The model under review builds one solid part; all positions refer to its coordinate system, in mm. Give positions to 0.01 mm unless a question says otherwise; leave off trailing zeros. Write each question's results on one line, items separated by ' | '. Start each with the question number.
Q1. Insertion check: pin 1 Ø1.3 at (x, z) = (3.5, -2.5) entering from +Y; pin 2 Ø6 at (x, z) = (7.5, 4.5) entering from -Y; pin 3 Ø1 at (x, z) = (-18, -8.5) entering from -Y. Each pin has a flat end and moves straight along its axis. Give the tip position at first contact, or say it passes through.
Q2. Wall thickness on L1, parallel to Y at x = -15.5, z = 5.5; L2, parallel to Y at x = -8, z = -5.75: over which ranges is each line inside the solid? List them lowest first. Write a range as [from, to].
Q3. Mouldability with a two-part tool opening along Z and no side actions: class faces 1 (the face through (16.507, 0.507, 8.229)), 2 (the face through (-15, 8, -4)), 3 (the face through (0, 4, 9.5)) as released by +Z, released by -Z, zero draft, split by the parting line, or undercut.
from build123d import *

# Parameters (mm, degrees)
SKETCH_1_W             = 37.6
SKETCH_1_H             = 19
EXTRUDE_1_DEPTH        = 8.1
SKETCH_3_R             = 0.75
CUT_EXTRUDE_1_DEPTH    = 0.1
PATTERN_LINEAR_1_COUNT = 3
PATTERN_LINEAR_1_PITCH = 12.7
CUT_EXTRUDE_4_DEPTH    = 28.929375217
CUT_EXTRUDE_5_DEPTH    = 40.618430055
EXTRUDE_3_DEPTH        = 2.5
EXTRUDE_3_DEPTH_BACK   = 1
SKETCH_7_R             = 0.25


with BuildPart() as part:
    # Эскиз1 → Бобышка-Вытянуть1 (new body)
    with BuildSketch(Plane(origin=(0, 0, 0), x_dir=(1, 0, 0), z_dir=(0, 1, 0))):
        Rectangle(SKETCH_1_W, SKETCH_1_H)
    extrude(amount=EXTRUDE_1_DEPTH)

    # Эскиз3 → Вырез-Вытянуть1 (cut)
    with BuildSketch(Plane(origin=(0, 8.1, 0), x_dir=(1, 0, 0), z_dir=(0, 1, 0))):
        with Locations(Location((-8.304984536, -7.1, 0), (0, 0, 270))):
            Circle(SKETCH_3_R)
        with BuildLine():
            Line((-16.613732692, -0.2), (-15.694010352, -0.2))
            Line((-15.694010352, -0.2), (-15.219253427, -0.887312434))
            Line((-15.219253427, -0.887312434), (-16.426812093, -7.1))
            Line((-16.426812093, -7.1), (-16.741799663, -7.1))
            ThreePointArc((-16.741799663, -7.1), (-17.513421017, -6.736082138), (-17.723428784, -5.909200972))
            Line((-17.723428784, -5.909200972), (-16.613732692, -0.2))
        make_face()
        Polygon((-15.447560185, -0.028936325), (-14.606711256, 0.75), (-10.084601751, 0.75), (-9.951753914, 0.611535824), (-9.389365278, 0.025371374), (-10.434703803, -0.75), (-14.949489793, -0.75), align=None)
        Polygon((-13.658315987, 5.6), (-13.366761329, 7.1), (-8.873187907, 7.1), (-9.164742565, 5.6), align=None)
        Polygon((-16.126812093, -7.1), (-15.835257435, -5.6), (-11.341684013, -5.6), (-11.633238671, -7.1), align=None)
        with BuildLine():
            Line((-8.405704285, 0.1), (-9.045218155, 0.1))
            Line((-9.045218155, 0.1), (-9.784090374, 0.870109138))
            Line((-9.784090374, 0.870109138), (-8.573187907, 7.1))
            Line((-8.573187907, 7.1), (-8.258200337, 7.1))
            ThreePointArc((-8.258200337, 7.1), (-7.486578983, 6.736082138), (-7.276571216, 5.909200972))
            Line((-7.276571216, 5.909200972), (-8.405704285, 0.1))
        make_face()
        with BuildLine():
            Line((-8.464015217, -0.2), (-9.087857218, -0.2))
            Line((-9.087857218, -0.2), (-9.189636199, -0.2))
            Line((-9.189636199, -0.2), (-10.127267632, -0.895480512))
            Line((-10.127267632, -0.895480512), (-11.333238671, -7.1))
            Line((-11.333238671, -7.1), (-10.629511556, -7.1))
            ThreePointArc((-10.629511556, -7.1), (-9.993429419, -6.871621354), (-9.647882436, -6.290799028))
            Line((-9.647882436, -6.290799028), (-8.464015217, -0.2))
        make_face()
        with BuildLine():
            Line((-16.555421761, 0.1), (-15.749822735, 0.1))
            Line((-15.749822735, 0.1), (-14.968967681, 0.823359864))
            Line((-14.968967681, 0.823359864), (-14.868695649, 0.916248759))
            Line((-14.868695649, 0.916248759), (-13.666761329, 7.1))
            Line((-13.666761329, 7.1), (-14.370488444, 7.1))
            ThreePointArc((-14.370488444, 7.1), (-15.006570581, 6.871621354), (-15.352117564, 6.290799028))
            Line((-15.352117564, 6.290799028), (-16.555421761, 0.1))
        make_face()
    cut_extrude_1 = extrude(amount=-CUT_EXTRUDE_1_DEPTH, mode=Mode.SUBTRACT)

    # Линейный массив1: Вырез-Вытянуть1 ×3
    with Locations(*[(i * PATTERN_LINEAR_1_PITCH, 0, 0) for i in range(1, PATTERN_LINEAR_1_COUNT)]):
        add(cut_extrude_1, mode=Mode.SUBTRACT)

    # Эскиз5 → Вырез-Вытянуть4 (cut, through all)
    with BuildSketch(Plane.XY.offset(9.5)):
        Polygon((-16.8, 0), (-16.222649731, 1), (16.222649731, 1), (16.8, 0), align=None)
    extrude(amount=-CUT_EXTRUDE_4_DEPTH, mode=Mode.SUBTRACT)

    # Эскиз6 → Вырез-Вытянуть5 (cut, through all)
    with BuildSketch(Plane(origin=(18.8, 0, 0), x_dir=(0, 0, -1), z_dir=(1, 0, 0))):
        Polygon((-7.5, 0), (-6.922649731, 1), (6.922649731, 1), (7.5, 0), align=None)
    extrude(amount=-CUT_EXTRUDE_5_DEPTH, mode=Mode.SUBTRACT)

    # Эскиз7 → Бобышка-Вытянуть3 (add, two sides: drawn at the far end of the back side and taken through both)
    with BuildSketch(Plane.XZ.offset(-1).offset(-EXTRUDE_3_DEPTH_BACK)):
        with Locations(Location((-1.27, -7.62, 0), (0, 0, 270))):
            Circle(SKETCH_7_R)
        with Locations(Location((-3.81, -7.62, 0), (0, 0, 270))):
            Circle(SKETCH_7_R)
        with Locations(Location((-6.35, -7.62, 0), (0, 0, 270))):
            Circle(SKETCH_7_R)
        with Locations((6.35, -7.62)):
            Circle(SKETCH_7_R)
        with Locations((3.81, -7.62)):
            Circle(SKETCH_7_R)
        with Locations((1.27, -7.62)):
            Circle(SKETCH_7_R)
        with Locations(Location((1.27, 7.62, 0), (0, 0, 270))):
            Circle(SKETCH_7_R)
        with Locations(Location((3.81, 7.62, 0), (0, 0, 270))):
            Circle(SKETCH_7_R)
        with Locations(Location((6.35, 7.62, 0), (0, 0, 270))):
            Circle(SKETCH_7_R)
        with Locations((-6.35, 7.62)):
            Circle(SKETCH_7_R)
        with Locations((-3.81, 7.62)):
            Circle(SKETCH_7_R)
        with Locations((-1.27, 7.62)):
            Circle(SKETCH_7_R)
    extrude(amount=EXTRUDE_3_DEPTH + EXTRUDE_3_DEPTH_BACK)


solid = part.part
Output:
1) pin 1: y = 8.1 | pin 2: y = 1 | pin 3: y = 0
2) L1: [1, 8.1] | L2: [1, 8]
3) face 1: zero draft | face 2: undercut | face 3: released by +Z
